Design review of the part built by this model. Coordinates are the model's own, in mm. A direction names the side the tool comes from. Give positions to 0.01 mm unless a question says otherwise; leave off trailing zeros. Loops run counter-clockwise (first coordinate to the right, second up) from the corner with the lowest first, then second, coordinate; pieces in that order, holes last. Notation, with made-up numbers: M 67,29.25 L 82,29.25 A18 ccw 82,43.25 Z; hole C 60,5 d7. An arc over 180 degrees is marked long. Use one line per item in the form item = value. Start each with the question number.
from build123d import *

# Parameters (mm, degrees)
RESSALTO_EXTRUS_O1_DEPTH = 2
ESBO_O2_R                = 3
ESBO_O2_R_2              = 1
CORTE_EXTRUS_O1_DEPTH    = 2
PADR_OCIRCULAR1_COUNT    = 18
ESBO_O3_W                = 16
ESBO_O3_H                = 1.561418551
CORTE_EXTRUS_O2_DEPTH    = 2


with BuildPart() as part:
    # Esboço1 → Ressalto-extrusão1 (new body)
    with BuildSketch(Plane(origin=(0, 0, 0), x_dir=(0, 0, -1), z_dir=(1, 0, 0))):
        with BuildLine():
            Line((-13, -71), (-13, -86))
            Line((-13, -86), (0, -86))
            Line((0, -86), (0, 15))
            ThreePointArc((0, 15), (-14.165790836, 4.932582487), (-9.316524238, -11.755950669))
            add(Edge.make_bspline(
                [(-9.316524238, -11.755950669), (-13, -71)],
                knots=[0, 0, 1, 1], degree=1))
        make_face()
    ressalto_extrus_o1 = extrude(amount=RESSALTO_EXTRUS_O1_DEPTH)

    # Espelhar1: Ressalto-extrusão1 across plane
    add(ressalto_extrus_o1.mirror(Plane(origin=(2, 15, 0), x_dir=(1, 0, 0), z_dir=(0, 0, 1))))

    # Esboço2 → Corte-extrusão1 (cut)
    with BuildSketch(Plane(origin=(2, 0, 0), x_dir=(0, 0, -1), z_dir=(1, 0, 0))):
        Circle(ESBO_O2_R)
        with Locations((0, -10)):
            Circle(ESBO_O2_R_2)
    corte_extrus_o1 = extrude(amount=-CORTE_EXTRUS_O1_DEPTH, mode=Mode.SUBTRACT)

    # PadrãoCircular1: Corte-extrusão1 ×18 about axis
    padr_ocircular1_axis = Axis((0, 0, 0), (1, 0, 0))
    for i in range(1, PADR_OCIRCULAR1_COUNT):
        add(corte_extrus_o1.rotate(padr_ocircular1_axis, i * 360 / PADR_OCIRCULAR1_COUNT), mode=Mode.SUBTRACT)

    # Esboço3 → Corte-extrusão2 (cut)
    with BuildSketch(Plane(origin=(2, 0, 0), x_dir=(0, 0, -1), z_dir=(1, 0, 0))):
        with BuildLine():
            Line((-4.922191444, -73), (4.922191444, -73))
            ThreePointArc((4.922191444, -73), (5.655263728, -72.680150738), (5.919390754, -71.925210052))
            Line((5.919390754, -71.925210052), (3.208172262, -35.775630155))
            ThreePointArc((3.208172262, -35.775630155), (2.257026545, -33.800783147), (0.216574332, -33))
            Line((0.216574332, -33), (-0.216574332, -33))
            ThreePointArc((-0.216574332, -33), (-2.257026545, -33.800783147), (-3.208172262, -35.775630155))
            Line((-3.208172262, -35.775630155), (-5.919390754, -71.925210052))
            ThreePointArc((-5.919390754, -71.925210052), (-5.655263728, -72.680150738), (-4.922191444, -73))
        make_face()
        with Locations((0, -81.719290725)):
            Rectangle(ESBO_O3_W, ESBO_O3_H)
    extrude(amount=-CORTE_EXTRUS_O2_DEPTH, mode=Mode.SUBTRACT)


solid = part.part
Q1. Take a section at B-B on x = 1. State how many separate pieces and enclosed holes the cut face has, plus the area to 3 significant figures.
Q2. Wall thickness on probe 1 along Y at (x, z) = (0.65, 0); probe 2 along Y at (x, z) = (1.05, -7); probe 3 along Y at (x, z) = (0.4, 2): over which ranges is each line inside the solid? List them lowest first.
Q3. For faces 1 (the flat face through (1.014, -53.597, 4.545)), 2 (the flat face through (1, -78, 13)), list the 3-axis set-ups (+Z, -Z, +X, -X, +Y, -Y) from which the entire face can be reached by the end or side of a thin tool; tool diameter is ignored.
Q4. Clearance check with a flat-ended pin moving along its axis: pin 1 Ø0.8 at (x, y) = (1.5, -81.5) entering from -Z. State where the tip first meets the part, or that it passes through.
Q5. The part is to be moulded in two halves that separate along Y. For faces 3 (the flat face through (1, -86, 0)), 4 (the cylindrical face through (1.01, 5.04, 9.66)), 5 (the flat face through (0, -35, -4)), say which applies: pulls with the +Y half, pulls with the -Y half, needs draft (parallel to the pull), parting line crosses it, or undercut.
Q6. Take a section at A-A on y = 5. Give the boundary of the cut face in (x, z), plus the area to 3 significant figures.
Response values:
q1.separate_pieces = 1
q1.enclosed_holes = 21
q1.area = 1,910 mm^2
q2.probe_1 = -86 to -82.5, -80.94 to -73, -33 to -11, -9 to -3, 3 to 9, 11 to 15
q2.probe_2 = -86 to -82.5, -80.94 to -8.48, -6.84 to 6.84, 8.48 to 13.27
q2.probe_3 = -86 to -82.5, -80.94 to -73, -33.59 to -2.24, 2.24 to 14.87
q3.face_1 = +X, -X
q3.face_2 = +Z, +X, -X, -Y
q4.pin_1 = -13
q5.face_3 = pulls with the -Y half
q5.face_4 = undercut
q5.face_5 = needs draft
q6.outline = M 0,-14.14 L 2,-14.14 L 2,-9.66 L 0,-9.66 Z; M 0,-7.66 L 2,-7.66 L 2,7.66 L 0,7.66 Z; M 0,9.66 L 2,9.66 L 2,14.14 L 0,14.14 Z
q6.area = 48.6 mm^2
